The listing builds one solid part. Answer for the finished solid, in the listing's coordinates (mm). Round coordinates to 2 decimals unless told otherwise and drop trailing zeros. Write each loop counter-clockwise with the first axis right and the second up, starting at its lowest first coordinate (ties: lowest second). Pieces come first, ordered by that corner, then holes. Notation, with made-up numbers: M -40,48.25 L -8,48.25 A16 cw -8,75.25 Z; hole C 38,37.25 d5. An arc over 180 degrees is marked long. One line per item, written item: value. Start each with the question number.
(1) Section A-A (x = 59) is taken. Determine the outline of the cut face in (y, z).
(2) Consider probe 1 along X at (y, z) = (6.25, -18); probe 2 along X at (y, z) = (0.5, -8); probe 3 along Z at (x, y) = (59.5, 1). Determine where each line is inside the solid, lowest interval first.
(3) Given P1, Ø15.5, axis at x = 23, z = -18, coming from the +Y side, flat-ended and moving along its own axis, determine where the tip first touches the part or whether it passes through.
(4) Section D-D (x = 137) is taken. Determine the outline of the cut face in (y, z).
(5) Section B-B (z = -18) is taken. Determine the outline of the cut face in (x, y), plus the area to 3 significant figures.
(6) Section C-C (y = 2.25) is taken. Determine the outline of the cut face in (x, z), plus the area to 3 significant figures.
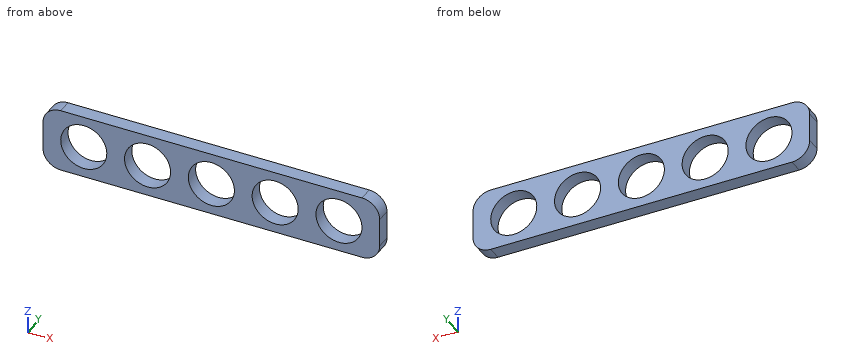
```python
from build123d import *

# Parameters (mm, degrees)
SKETCH5_W           = 190
SKETCH5_H           = 36
BOSS_EXTRUDE1_DEPTH = 8
SKETCH6_R           = 13
SKETCH6_R_2         = 12.99768992
CUT_EXTRUDE1_DEPTH  = 8
FILLET2_R           = 10


with BuildPart() as part:
    # Sketch5 → Boss-Extrude1 (new body)
    with BuildSketch(Plane(origin=(0, 0, 0), x_dir=(1, 0, 0), z_dir=(0, 1, 0))):
        with Locations((95, 18)):
            Rectangle(SKETCH5_W, SKETCH5_H)
    extrude(amount=BOSS_EXTRUDE1_DEPTH)

    # Sketch6 → Cut-Extrude1 (cut)
    with BuildSketch(Plane(origin=(0, 8, 0), x_dir=(1, 0, 0), z_dir=(0, 1, 0))):
        with Locations(Location((23, 18, 0), (0, 0, 270))):
            Circle(SKETCH6_R)
        with Locations(Location((59, 18, 0), (0, 0, 270))):
            Circle(SKETCH6_R)
        with Locations(Location((95.004620161, 18, 0), (0, 0, 270))):
            Circle(SKETCH6_R)
        with Locations(Location((131.004620161, 18, 0), (0, 0, 270))):
            Circle(SKETCH6_R)
        with Locations(Location((167.00231008, 18, 0), (0, 0, 270))):
            Circle(SKETCH6_R_2)
    extrude(amount=-CUT_EXTRUDE1_DEPTH, mode=Mode.SUBTRACT)

    # Fillet2
    fillet2_edges = [part.edges().sort_by_distance(p)[0] for p in [
        (0, 4, -36),
        (190, 4, -36),
        (190, 4, 0),
        (0, 4, 0),
    ]]
    fillet(fillet2_edges, radius=FILLET2_R)


solid = part.part
```
Recorded:
1. outline: M 0,-36 L 8,-36 L 8,-31 L 0,-31 Z; M 0,-5 L 8,-5 L 8,0 L 0,0 Z
2. probe 1: x = 0 to 10, 36 to 46, 72 to 82, 108 to 118, 144 to 154, 180 to 190
2. probe 2: x = 0.2 to 14.69, 31.31 to 50.69, 67.31 to 86.7, 103.31 to 122.7, 139.31 to 158.7, 175.31 to 189.8
2. probe 3: z = -36 to -30.99, -5.01 to 0
3. P1: passes through
4. outline: M 0,-36 L 8,-36 L 8,-29.53 L 0,-29.53 Z; M 0,-6.47 L 8,-6.47 L 8,0 L 0,0 Z
5. outline: M 0,0 L 10,0 L 10,8 L 0,8 Z; M 36,0 L 46,0 L 46,8 L 36,8 Z; M 72,0 L 82,0 L 82,8 L 72,8 Z; M 108,0 L 118,0 L 118,8 L 108,8 Z; M 144,0 L 154,0 L 154,8 L 144,8 Z; M 180,0 L 190,0 L 190,8 L 180,8 Z
5. area: 480 mm2
6. outline: M 0,-26 A10 ccw 10,-36 L 180,-36 A10 ccw 190,-26 L 190,-10 A10 ccw 180,0 L 10,0 A10 ccw 0,-10 Z; hole C 23,-18 d26; hole C 59,-18 d26; hole C 95,-18 d26; hole C 131,-18 d26; hole C 167,-18 d26
6. area: 4,100 mm2
